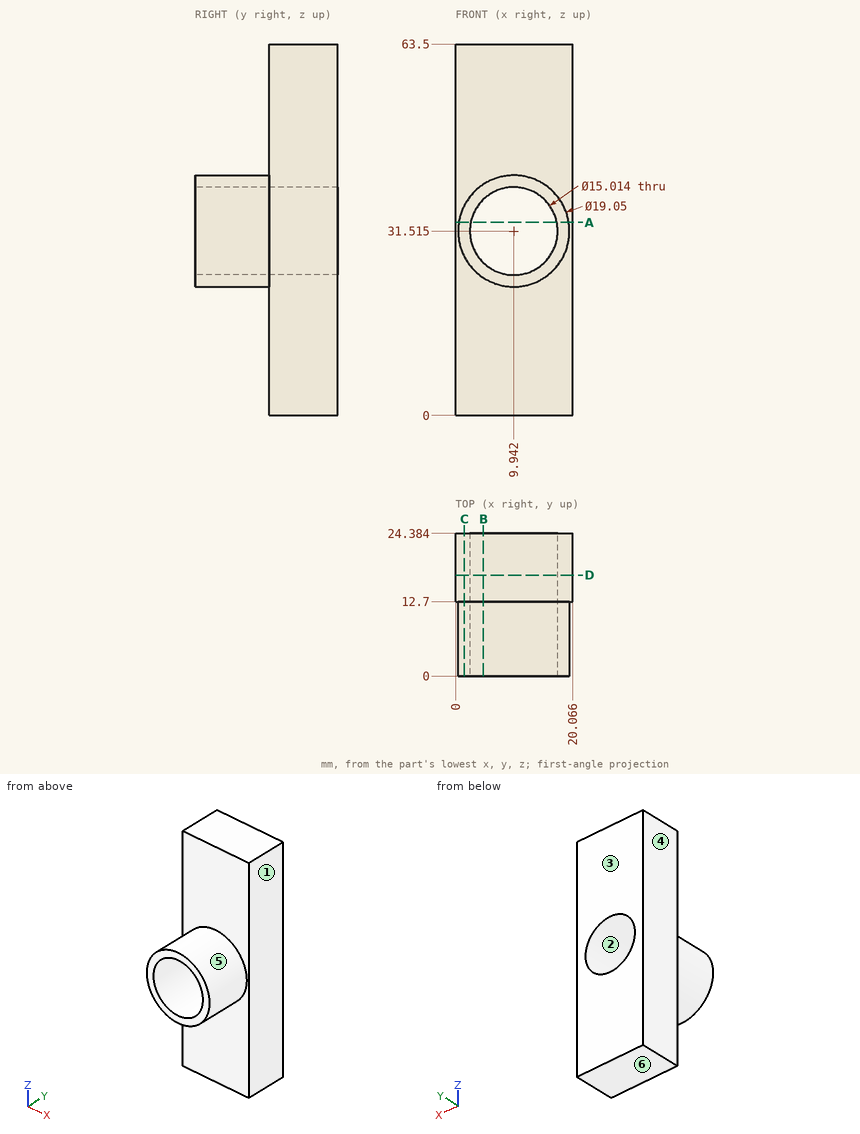
Part print with two shaded views. Sizes in mm from the minimum x, y, z corner. A direction names the side the tool comes from. Coordinates: 2 decimals unless noted, no trailing zeros. Write each loop counter-clockwise with the first axis right and the second up, starting at its lowest first coordinate (ties: lowest second). Pieces come first, ordered by that corner, then holes. Notation, with made-up numbers: (43, -36) - (65, -36) arc R36 cw to (65, 0) - close; hole circle Ø11 at (-18.5, 2). An arc over 180 degrees is marked (long way). Put each result on its own line as item: value.
1. Flat gauge pins, fed straight in: pin 1 Ø12 at (x, y) = (2, 4) entering from +Z; pin 2 Ø8 at (x, y) = (5, 7) entering from -Z; pin 3 Ø3 at (x, y) = (16.5, 11) entering from +Z (1 decimal). Where does each tip first touch, or does it go through?
Final values:
pin 1: stops at z = 40.84
pin 2: stops at z = 22.04
pin 3: stops at z = 39.6
2. Two-plate mould, pull along X, no slides. Class the marked faces 1, 2, 3 and 4: +X half, -X half, draft (parallel to the pull), parting line (faces both ways), or undercut.
Final values:
face 1: +X half
face 2: undercut
face 3: draft
face 4: -X half
3. Band-saw the part on D-D (y = 17.25). Write the cut outline in (x, z) (1 decimal).
Final values:
outline: (0, 0) - (20.1, 0) - (20.1, 63.5) - (0, 63.5) - close; hole circle Ø15 at (9.9, 31.5)
4. Band-saw the part on B-B (x = 4.75). Write the cut outline in (y, z), then the cut area to 3 significant figures.
Final values:
outline: (0, 23.53) - (12.7, 23.53) - (12.7, 0) - (24.38, 0) - (24.38, 26.09) - (0, 26.09) - close; (0, 36.94) - (24.38, 36.94) - (24.38, 63.5) - (12.7, 63.5) - (12.7, 39.5) - (0, 39.5) - close
area: 680 mm²
5. Band-saw the part on A-A (z = 33). Write the cut outline in (x, y).
Final values:
outline: (0, 12.7) - (0.53, 12.7) - (0.53, 0) - (2.58, 0) - (2.58, 24.38) - (0, 24.38) - close; (17.3, 0) - (19.35, 0) - (19.35, 12.7) - (20.07, 12.7) - (20.07, 24.38) - (17.3, 24.38) - close
6. Probe line 1 along Z through (x, y) = (10, 18); line 2 along Y through (x, z) = (10.5, 18); line 3 along Z through (x, y) = (14.75, 5). List the from-to ranges inside material, lowest first. Write a range as [from, to].
Final values:
line 1: z = [0, 24.01], [39.02, 63.5]
line 2: y = [12.7, 24.38]
line 3: z = [23.29, 25.75], [37.28, 39.74]
7. 3-axis set-ups, long thin cutter, end or side, ignore diameter. For the marked faces 5 and 6: which of +Z, -Z, +X, -X, +Y, -Y reach the whole face in a straight line?
Final values:
face 5: -Y
face 6: -Z, +X, -X, +Y, -Y
8. Band-saw the part on C-C (x = 1.5). Write the cut outline in (y, z).
Final values:
outline: (0, 27.1) - (12.7, 27.1) - (12.7, 0) - (24.38, 0) - (24.38, 63.5) - (12.7, 63.5) - (12.7, 35.93) - (0, 35.93) - close
